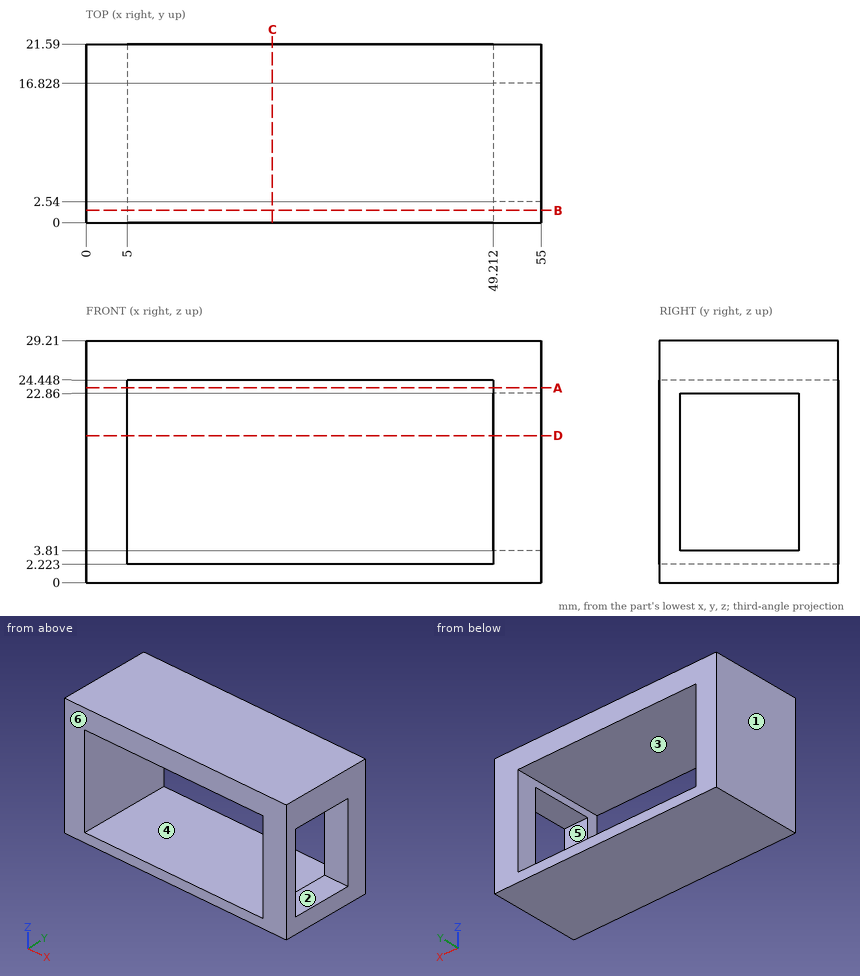
Verification items for this drawing (mm, ordinates from the low corner). A direction names the side the tool comes from. Coordinates: 2 decimals unless noted, no trailing zeros. Order: outer loops, then holes, each group sorted by start corner. A loop starts at its lowest first (then second) coordinate and runs counter-clockwise, first axis right, second up. Notation, with made-up numbers: M -2,36.5 L 15,36.5 A12 cw 15,41.5 Z; hole C 8.25,40 d10. An arc over 180 degrees is marked long. Answer as a JSON object with one key per item and string values.
Q1. Cross-section at A-A on z = 23.5. Record the cut outline in (x, y).
Results are:
{"outline": "M 0,0 L 5,0 L 5,21.59 L 0,21.59 Z; M 49.21,0 L 55,0 L 55,21.59 L 49.21,21.59 Z"}
Q2. Release check for a two-part mould opening along Y. For the marked faces 4, 5 and 6 record: released by +Y, released by -Y, zero draft, split by the parting line, or undercut.
Results are:
{"face 4": "zero draft", "face 5": "undercut", "face 6": "released by -Y"}
Q3. Cross-section at B-B on y = 1.5. Record the cut outline in (x, z), and give its area (3 significant figures).
Results are:
{"outline": "M 0,0 L 55,0 L 55,29.21 L 0,29.21 Z; hole M 5,2.22 L 49.21,2.22 L 49.21,24.45 L 5,24.45 Z", "area": "624 mm²"}
Q4. Cross-section at D-D on z = 17.75. Record the cut outline in (x, y), and give its area (3 significant figures).
Results are:
{"outline": "M 0,0 L 5,0 L 5,21.59 L 0,21.59 Z; M 49.21,0 L 55,0 L 55,2.54 L 49.21,2.54 Z; M 49.21,16.83 L 55,16.83 L 55,21.59 L 49.21,21.59 Z", "area": "150 mm²"}
Q5. Depth check by flat-ended pin: pin 1 Ø8 at (x, y) = (12.5, 14.5) entering from -Z. Enter the tip coordinate at first touch or a pass-through.
Results are:
{"pin 1": "stops at z = 0"}
Q6. Tool access check on the marked faces 1, 2 and 3. Record the directions out of +Z, -Z, +X, -X, +Y, -Y that give a thin tool (end or side, any length) a straight path to the whole face; none if there is none.
Results are:
{"face 1": "+Z, -Z, -X, +Y, -Y", "face 2": "+X", "face 3": "+Y, -Y"}
Q7. Scan lines: line 1 (Z direction, x = 51.5, y = 9.25); line 2 (Z direction, x = 13, y = 9.75); line 3 (X direction, y = 1.25, z = 18.25). Record each from-to range of solid material in increasing order.
Results are:
{"line 1": "z = 0 to 3.81, 22.86 to 29.21", "line 2": "z = 0 to 2.22, 24.45 to 29.21", "line 3": "x = 0 to 5, 49.21 to 55"}
Q8. Cross-section at C-C on x = 22.5. Record the cut outline in (y, z).
Results are:
{"outline": "M 0,0 L 21.59,0 L 21.59,2.22 L 0,2.22 Z; M 0,24.45 L 21.59,24.45 L 21.59,29.21 L 0,29.21 Z"}
